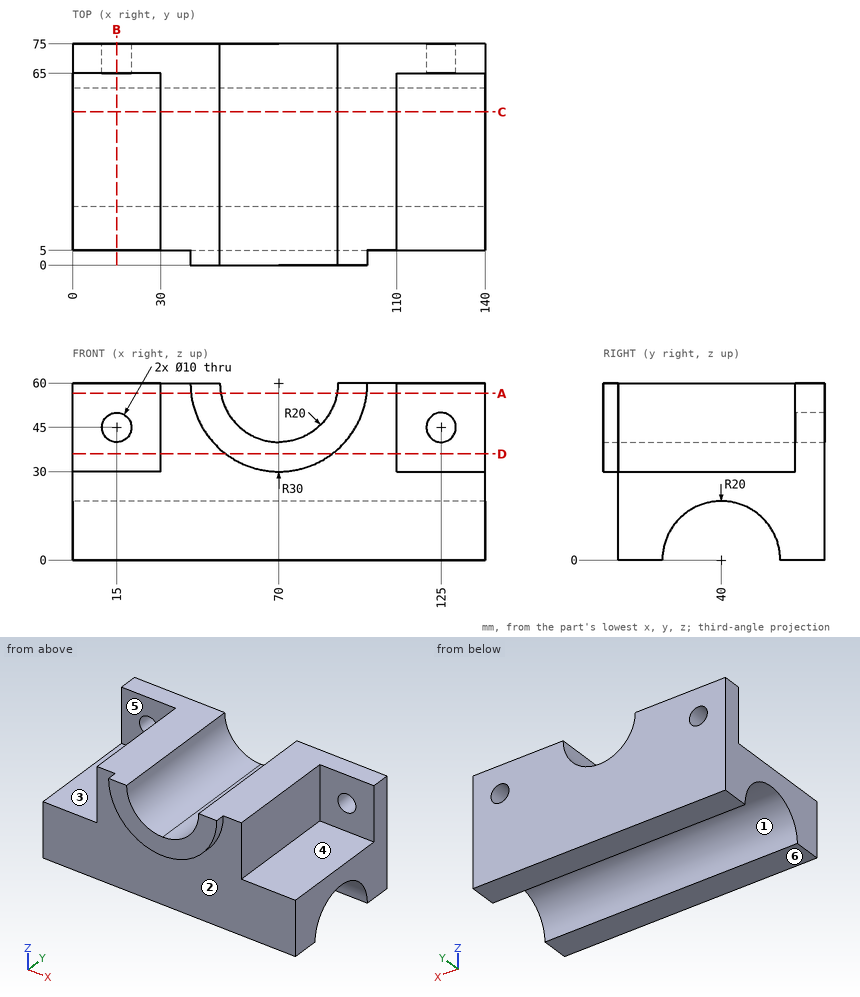
The drawing under review shows one solid part. Ordinate dimensions are in mm from its lowest x, y, z. A direction names the side the tool comes from. Coordinates: 2 decimals unless noted, no trailing zeros. Write each loop counter-clockwise with the first axis right and the second up, starting at its lowest first coordinate (ties: lowest second). Pieces come first, ordered by that corner, then holes.
1) Add section C-C (y = 52). Write out the cut boundary in (x, z).
2) To check wall thickness, follow L1, parallel to Z at x = 125, y = 71.5; L2, parallel to Y at x = 25, z = 40.5; L3, parallel to X at y = 60, z = 32. State the ranges of each line that lie inside material, in increasing order.
3) Insertion check: pin 1 (2 mm diameter, centred on y = 24, z = 48, fed in from -X); pin 2 (5 mm diameter, centred on y = 28, z = 33.5, fed in from +X); pin 3 (6 mm diameter, centred on x = 107, z = 30.5, fed in from -Y). Each pin has a flat end and moves straight along its axis. Give the tip position at first contact, or say it passes through.
4) Add section D-D (z = 36). Write out the cut boundary in (x, y).
5) Mouldability with a two-part tool opening along Y and no side actions: class the marked faces 1, 2 and 3 as +Y half, -Y half, draft (parallel to the pull), parting line (faces both ways), or undercut.
6) Add section B-B (x = 15). Write out the cut boundary in (y, z), plus the area to 3 significant figures.
7) Add section A-A (z = 56.5). Write out the cut boundary in (x, y).
8) Machinability: for the marked faces 4, 5 and 6, which of the approach directions +Z, -Z, +X, -X, +Y, -Y give a long, thin tool a straight path to every point of the face, cutting with its end or side? Answer none if there is none.
Check result:
1. outline: (0, 16) - (140, 16) - (140, 30) - (110, 30) - (110, 60) - (90, 60) arc R20 cw to (50, 60) - (30, 60) - (30, 30) - (0, 30) - close
2. L1: z = 0 to 40, 50 to 60
2. L2: y = 65 to 75
2. L3: x = 30 to 110
3. pin 1: stops at x = 30
3. pin 2: stops at x = 110
3. pin 3: stops at y = 5
4. outline: (0, 65) - (30, 65) - (30, 5) - (52, 5) - (52, 0) - (88, 0) - (88, 5) - (110, 5) - (110, 65) - (140, 65) - (140, 75) - (0, 75) - close
5. face 1: undercut
5. face 2: -Y half
5. face 3: draft
6. outline: (5, 0) - (20, 0) arc R20 cw to (60, 0) - (75, 0) - (75, 40) - (65, 40) - (65, 30) - (5, 30) - close; (65, 50) - (75, 50) - (75, 60) - (65, 60) - close
6. area: 1,670 mm2
7. outline: (0, 65) - (30, 65) - (30, 5) - (40.2, 5) - (40.2, 0) - (50.31, 0) - (50.31, 75) - (0, 75) - close; (89.69, 0) - (99.8, 0) - (99.8, 5) - (110, 5) - (110, 65) - (140, 65) - (140, 75) - (89.69, 75) - close
8. face 4: +Z, +X, -Y
8. face 5: +Z, -X, -Y
8. face 6: -Z, +X, -X, +Y, -Y
